from build123d import *

# Parameters (mm, degrees)
SKETCH_2_R          = 2.55
EXTRUDE_1_DEPTH     = 120
SKETCH_3_R          = 3
CUT_EXTRUDE_1_DEPTH = 123.065556157


with BuildPart() as part:
    # 草图2 → 凸台-拉伸1 (new body)
    with BuildSketch(Plane.XY):
        with BuildLine():
            Line((-3.9, 2.839339828), (-6.560660172, 5.5))
            Line((-6.560660172, 5.5), (-8.2, 5.5))
            Line((-8.2, 5.5), (-8.2, 3.1))
            Line((-8.2, 3.1), (-9.45, 3.1))
            Line((-9.45, 3.1), (-9.45, 3.65))
            Line((-9.45, 3.65), (-10, 3.65))
            Line((-10, 3.65), (-10, 8.5))
            ThreePointArc((-10, 8.5), (-9.560660172, 9.560660172), (-8.5, 10))
            Line((-8.5, 10), (-3.65, 10))
            Line((-3.65, 10), (-3.65, 9.45))
            Line((-3.65, 9.45), (-3.1, 9.45))
            Line((-3.1, 9.45), (-3.1, 8.2))
            Line((-3.1, 8.2), (-5.5, 8.2))
            Line((-5.5, 8.2), (-5.5, 6.560660172))
            Line((-5.5, 6.560660172), (-2.839339828, 3.9))
            Line((-2.839339828, 3.9), (2.839339828, 3.9))
            Line((2.839339828, 3.9), (5.5, 6.560660172))
            Line((5.5, 6.560660172), (5.5, 8.2))
            Line((5.5, 8.2), (3.1, 8.2))
            Line((3.1, 8.2), (3.1, 9.45))
            Line((3.1, 9.45), (3.65, 9.45))
            Line((3.65, 9.45), (3.65, 10))
            Line((3.65, 10), (8.5, 10))
            ThreePointArc((8.5, 10), (9.560660172, 9.560660172), (10, 8.5))
            Line((10, 8.5), (10, 3.65))
            Line((10, 3.65), (9.45, 3.65))
            Line((9.45, 3.65), (9.45, 3.1))
            Line((9.45, 3.1), (8.2, 3.1))
            Line((8.2, 3.1), (8.2, 5.5))
            Line((8.2, 5.5), (6.560660172, 5.5))
            Line((6.560660172, 5.5), (3.9, 2.839339828))
            Line((3.9, 2.839339828), (3.9, -2.839339828))
            Line((3.9, -2.839339828), (6.560660172, -5.5))
            Line((6.560660172, -5.5), (8.2, -5.5))
            Line((8.2, -5.5), (8.2, -3.1))
            Line((8.2, -3.1), (9.45, -3.1))
            Line((9.45, -3.1), (9.45, -3.65))
            Line((9.45, -3.65), (10, -3.65))
            Line((10, -3.65), (10, -8.5))
            ThreePointArc((10, -8.5), (9.560660172, -9.560660172), (8.5, -10))
            Line((8.5, -10), (3.65, -10))
            Line((3.65, -10), (3.65, -9.45))
            Line((3.65, -9.45), (3.1, -9.45))
            Line((3.1, -9.45), (3.1, -8.2))
            Line((3.1, -8.2), (5.5, -8.2))
            Line((5.5, -8.2), (5.5, -6.560660172))
            Line((5.5, -6.560660172), (2.839339828, -3.9))
            Line((2.839339828, -3.9), (-2.839339828, -3.9))
            Line((-2.839339828, -3.9), (-5.5, -6.560660172))
            Line((-5.5, -6.560660172), (-5.5, -8.2))
            Line((-5.5, -8.2), (-3.1, -8.2))
            Line((-3.1, -8.2), (-3.1, -9.45))
            Line((-3.1, -9.45), (-3.65, -9.45))
            Line((-3.65, -9.45), (-3.65, -10))
            Line((-3.65, -10), (-8.5, -10))
            ThreePointArc((-8.5, -10), (-9.560660172, -9.560660172), (-10, -8.5))
            Line((-10, -8.5), (-10, -3.65))
            Line((-10, -3.65), (-9.45, -3.65))
            Line((-9.45, -3.65), (-9.45, -3.1))
            Line((-9.45, -3.1), (-8.2, -3.1))
            Line((-8.2, -3.1), (-8.2, -5.5))
            Line((-8.2, -5.5), (-6.560660172, -5.5))
            Line((-6.560660172, -5.5), (-3.9, -2.839339828))
            Line((-3.9, -2.839339828), (-3.9, 2.839339828))
        make_face()
        Circle(SKETCH_2_R, mode=Mode.SUBTRACT)
    extrude(amount=EXTRUDE_1_DEPTH)

    # 草图3 → 切除-拉伸1 (cut, through all)
    with BuildSketch(Plane(origin=(10, 0, 0), x_dir=(0, 0, -1), z_dir=(1, 0, 0))):
        with Locations(Location((-57.5, 0, 0), (0, 0, 71.16400384))):
            Circle(SKETCH_3_R)
        with Locations((-302.5, 0)):
            Circle(SKETCH_3_R)
    extrude(amount=-CUT_EXTRUDE_1_DEPTH, mode=Mode.SUBTRACT)


solid = part.part
Input: part model. Units: mm. Frame: model coordinates. A direction names the side the tool comes from. Coordinates: 2 decimals unless noted, no trailing zeros. Loops run counter-clockwise (first coordinate to the right, second up) from the corner with the lowest first, then second, coordinate; pieces in that order, holes last.
Q1. Draft query along X for faces 4 (the face through (8.2, 4, 59)), 5 (the face through (-6, 10, 59)), 6 (the face through (-10, 6, 59)). Return one class per face: +X half, -X half, draft (parallel to the pull), parting line (faces both ways), or undercut.
Q2. Set-up query: faces 1 (the face through (8.2, -4, 59)), 2 (the face through (-3.9, 0, 28)), 3 (the face through (0, -3.9, 59)). Return all of +Z, -Z, +X, -X, +Y, -Y with unobstructed straight access to the full face (end or side cutting, diameter ignored); none if empty.
Q3. Cut plane A-A (y = 0). Output: boundary loops of the cut face in (x, z).
Q4. Material intervals for line 1 (X direction, y = 0, z = 43.5); line 2 (X direction, y = -4.5, z = 45), sorted ascending.
Q5. Contact query for flat-ended pins moving along their axis: pin 1 (3 mm diameter, centred on y = -0.5, z = 35, fed in from -X); pin 2 (4.5 mm diameter, centred on y = -1, z = 41, fed in from +X); pin 3 (0.6 mm diameter, centred on x = -10, z = 79.5, fed in from +Y). Output: stop coordinate, or through.
Working result:
1. face 4: undercut
1. face 5: draft
1. face 6: -X half
2. face 1: +Z, -Z
2. face 2: +Z, -Z, -X
2. face 3: +Z, -Z, -Y
3. outline: (-3.9, 0) - (-2.55, 0) - (-2.55, 54.5) - (-3.9, 54.5) - close; (-3.9, 60.5) - (-2.55, 60.5) - (-2.55, 120) - (-3.9, 120) - close; (2.55, 0) - (3.9, 0) - (3.9, 54.5) - (2.55, 54.5) - close; (2.55, 60.5) - (3.9, 60.5) - (3.9, 120) - (2.55, 120) - close
4. line 1: x = -3.9 to -2.55, 2.55 to 3.9
4. line 2: x = -10 to -8.2, -5.56 to -3.44, 3.44 to 5.56, 8.2 to 10
5. pin 1: stops at x = -3.9
5. pin 2: stops at x = 9.45
5. pin 3: stops at y = 9.4
